Here's how the part is built. I have some questions about the finished solid (model axes, mm). Face numbers are marked on the shaded views. A direction names the side the tool comes from. Coordinates: 2 decimals unless noted, no trailing zeros. Write each loop counter-clockwise with the first axis right and the second up, starting at its lowest first coordinate (ties: lowest second). Pieces come first, ordered by that corner, then holes. Notation, with made-up numbers: M 19.5,-4.75 L 57.5,-4.75 A30 ccw 57.5,20.25 Z; hole C -18,62.25 d10. An arc over 180 degrees is marked long. Write each question's results on one line, items separated by ' | '. Start each with the question number.
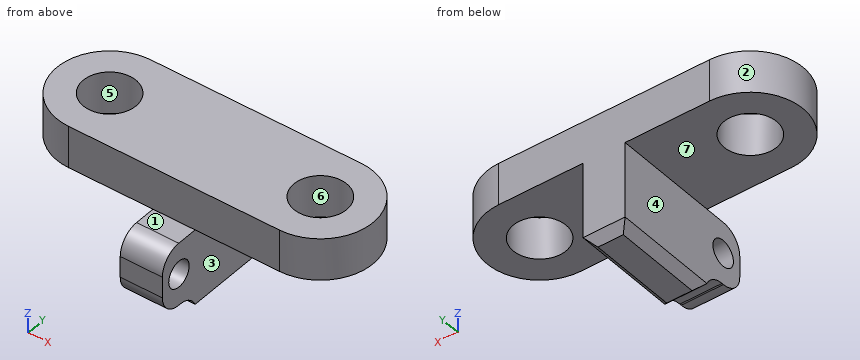
from build123d import *

# Parameters (mm, degrees)
F0_R         = 3.175
F1_DEPTH     = 22.86
F2_W         = 6.35
F2_H         = 6.35
F2_W_2       = 6.7925655007
F3_DEPTH     = 25.4
F5_DEPTH     = 25.4
F6_SIZE      = 1.016
F7_W         = 5.08
F7_H         = 7.62
F8_DEPTH     = 5.08
F9_R         = 1.5875
F10_DEPTH    = 25.4
F11_T1_DEPTH = 5.08
F11_T3_DEPTH = 17.78
F11_T5_DEPTH = 17.78


# Not quite as in the source:
# - a fillet or chamfer that OpenCascade refuses, or shapes differently, is made with other operations: its cross-section is extruded or revolved along the edge and cut away or added


with BuildPart() as f1:
    # F0 (on Top) → F1 (new body)
    with BuildSketch(Plane.XY):
        with BuildLine():
            Line((0, 6.35), (-25.4, 6.35))
            ThreePointArc((-25.4, 6.35), (-31.75, 0), (-25.4, -6.35))
            Line((-25.4, -6.35), (0, -6.35))
            ThreePointArc((0, -6.35), (6.35, 0), (0, 6.35))
        make_face()
        with Locations((-25.4, 0)):
            Circle(F0_R, mode=Mode.SUBTRACT)
        with BuildLine():
            ThreePointArc((3.175, 0), (0, -3.175), (-3.175, 0))
            ThreePointArc((-3.175, 0), (0, 3.175), (3.175, 0))
        make_face(mode=Mode.SUBTRACT)
    extrude(amount=F1_DEPTH)

    # F2 (on face) → F3 (cut)
    with BuildSketch(Plane(origin=(0, 6.35, 0), x_dir=(-1, 0, 0), z_dir=(0, 1, 0))):
        with Locations((-3.175, 8.255)):
            Rectangle(F2_W, F2_H)
        with Locations((28.7962827504, 14.605)):
            Rectangle(F2_W_2, F2_H)
        with Locations((28.7962827504, 8.255)):
            Rectangle(F2_W_2, F2_H)
        with Locations((3.175, 8.255)):
            Rectangle(F2_W, F2_H)
        with Locations((3.175, 14.605)):
            Rectangle(F2_W, F2_H)
        with Locations((22.225, 14.605)):
            Rectangle(F2_W, F2_H)
        with Locations((22.225, 8.255)):
            Rectangle(F2_W, F2_H)
        with Locations((-3.175, 14.605)):
            Rectangle(F2_W, F2_H)
    extrude(amount=-F3_DEPTH, mode=Mode.SUBTRACT)

    # F4 (on face) → F5 (cut)
    with BuildSketch(Plane(origin=(0, 6.35, 0), x_dir=(-1, 0, 0), z_dir=(0, 1, 0))):
        Polygon((10.16, 17.78), (6.35, 17.78), (-14.3396928906, 11.8959285319), (-15.9743130207, -5.6489794515), (34.4809181988, -5.6489794515), (40.5834950507, 3.3959113061), (19.05, 17.78), (15.24, 17.78), (15.24, 7.62), (10.16, 7.62), align=None)
    extrude(amount=-F5_DEPTH, mode=Mode.SUBTRACT)

    # F6
    f6_edges = [f1.edges().sort_by_distance(p)[0] for p in [
        (-15.24, 0, 7.62),
        (-10.16, 0, 7.62),
        (-12.7, -6.35, 7.62),
        (-12.7, 6.35, 7.62),
    ]]
    chamfer(f6_edges, length=F6_SIZE)

    # F7 (on face) → F8 (join)
    with BuildSketch(Plane.XZ.offset(6.35)):
        with Locations((-12.7, 13.97)):
            Rectangle(F7_W, F7_H)
    extrude(amount=F8_DEPTH)

    # F9 (on face) → F10 (cut)
    with BuildSketch(Plane(origin=(-15.24, 0, 0), x_dir=(0, -1, 0), z_dir=(-1, 0, 0))):
        with Locations((8.8569838554, 13.97)):
            Circle(F9_R)
    extrude(amount=-F10_DEPTH, mode=Mode.SUBTRACT)

    # F11: fillet of radius 2.54 on 3 edges, made by hand

    # F11_s2 → F11_t1 (join)
    with BuildSketch(Plane.YZ.offset(-15.24)):
        with BuildLine():
            ThreePointArc((-8.677948453, 10.16), (-7.286733157, 9.7451164674), (-6.35, 8.636))
            Line((-6.35, 8.636), (-6.35, 10.16))
            Line((-6.35, 10.16), (-8.677948453, 10.16))
        make_face()
    extrude(amount=F11_T1_DEPTH)

    # F11_s4 → F11_t3 (cut)
    with BuildSketch(Plane.YZ.offset(-21.59)):
        with BuildLine():
            ThreePointArc((-8.89, 17.78), (-10.6860512242, 17.0360512242), (-11.43, 15.24))
            Line((-11.43, 15.24), (-11.43, 17.78))
            Line((-11.43, 17.78), (-8.89, 17.78))
        make_face()
    extrude(amount=F11_T3_DEPTH, mode=Mode.SUBTRACT)

    # F11_s6 → F11_t5 (cut)
    with BuildSketch(Plane.YZ.offset(-21.59)):
        with BuildLine():
            ThreePointArc((-8.89, 10.16), (-10.6860512242, 10.9039487758), (-11.43, 12.7))
            Line((-11.43, 12.7), (-11.43, 10.16))
            Line((-11.43, 10.16), (-8.89, 10.16))
        make_face()
    extrude(amount=F11_T5_DEPTH, mode=Mode.SUBTRACT)


solid = f1.part
1) Please list where these lines run through material, in increasing order: line 1 (X direction, y = -0.5, z = 21); line 2 (Y direction, x = -25.4, z = 21.45) (3 decimals); line 3 (X direction, y = -2, z = 18.5). Write a range as [from, to].
2) I want a section at B-B, the plane z = 13.97. Write out the boundary of the cut face in (x, y), then the cut area to 3 significant figures.
3) I want a section at C-C, the plane x = -23. Write out the boundary of the cut face in (y, z).
4) We'd pull the mould along X, two halves only. Please class the marked faces 4, 5, 6 and 7: pulls with the +X half, pulls with the -X half, needs draft (parallel to the pull), parting line crosses it, or undercut.
5) For the marked faces 1, 2 and 3, which set-ups out of +Z, -Z, +X, -X, +Y, -Y let a thin tool reach every point of the face, with its end or its side?
6) For pin 1 Ø6 at (y, z) = (0, 11.5) entering from -X; pin 2 Ø6.5 at (x, y) = (-2.5, -3) entering from -Z; pin 3 Ø1.5 at (x, z) = (-12.5, 21) entering from -Y; pin 4 Ø1.5 at (x, z) = (-21.5, 16.5) entering from -Y, each with a flat end and sliding along its axis, tell me the tip position at first contact or that it passes through.
7) I want a section at A-A, the plane y = 0. Write out the boundary of the cut face in (x, z) (3 decimals).
8) I want a section at D-D, the plane z = 20. Write out the boundary of the cut face in (x, y) (3 decimals).
Output:
1) line 1: x = [-31.73, -28.54], [-22.26, -3.14], [3.14, 6.33] | line 2: y = [-6.35, -3.175], [3.175, 6.35] | line 3: x = [-31.43, -27.87], [-22.93, -2.47], [2.47, 6.03]
2) outline: M -15.24,-11.43 L -10.16,-11.43 L -10.16,-10.44 L -15.24,-10.44 Z; M -15.24,-7.27 L -10.16,-7.27 L -10.16,6.35 L -15.24,6.35 Z | area: 74.2 mm2
3) outline: M -6.35,17.78 L -2.08,17.78 L -2.08,22.86 L -6.35,22.86 Z; M 2.08,17.78 L 6.35,17.78 L 6.35,22.86 L 2.08,22.86 Z
4) face 4: pulls with the -X half | face 5: undercut | face 6: undercut | face 7: needs draft
5) face 1: +Z, +X, -X, -Y | face 2: +Z, -Z, -X | face 3: -Z, +X, +Y, -Y
6) pin 1: stops at x = -15.24 | pin 2: stops at z = 17.78 | pin 3: stops at y = -6.35 | pin 4: passes through
7) outline: M -31.75,17.78 L -28.575,17.78 L -28.575,22.86 L -31.75,22.86 Z; M -22.225,17.78 L -15.24,17.78 L -15.24,8.636 L -14.224,7.62 L -11.176,7.62 L -10.16,8.636 L -10.16,17.78 L -3.175,17.78 L -3.175,22.86 L -22.225,22.86 Z; M 3.175,17.78 L 6.35,17.78 L 6.35,22.86 L 3.175,22.86 Z
8) outline: M -25.4,-6.35 L 0,-6.35 A6.35 ccw 0,6.35 L -25.4,6.35 A6.35 ccw Z; hole C -25.4,0 d6.35; hole C 0,0 d6.35
